For this review, take the finished solid that the model builds, in its own axes (mm). Face numbers are marked on the shaded views. Give positions to 0.01 mm unless a question says otherwise; leave off trailing zeros. Loops run counter-clockwise (first coordinate to the right, second up) from the corner with the lowest first, then second, coordinate; pieces in that order, holes last. Notation, with made-up numbers: M 30,82.25 L 65,82.25 A28 cw 65,105.25 Z; hole C 21,33.25 d5. An arc over 180 degrees is marked long. Use CSV: the item, a comma, the result in double quotes. Start each with the question number.
1. Take a section at C-C, the plane y = -357. Write out the cut boundary in (x, z).
2. To check wall thickness, follow line 1 (X direction, y = -164, z = 37.5); line 2 (X direction, y = -377.5, z = 65); line 3 (Y direction, x = -47.5, z = 100.5). State the ranges of each line that lie inside material, in increasing order. Write a range as [from, to].
3. Take a section at D-D, the plane x = -31. Write out the cut boundary in (y, z).
4. Take a section at B-B, the plane x = 20.5. Write out the cut boundary in (y, z).
5. Take a section at A-A, the plane z = 43. Write out the cut boundary in (x, y), and give its area (3 significant figures).
6. Insertion check: P1, Ø3, axis at x = -8.5, y = -187.5, coming from the +Z side; P2, Ø2, axis at y = -120.5, z = 373.5, coming from the -X side; P3, Ø5, axis at y = -248.5, z = 284, coming from the +X side. Each pin has a flat end and moves straight along its axis. Give the tip position at first contact, or say it passes through.
7. The part is to be moulded in two halves that separate along X. For the marked faces 1, 2, 3 and 4, say which applies: pulls with the +X half, pulls with the -X half, needs draft (parallel to the pull), parting line crosses it, or undercut.
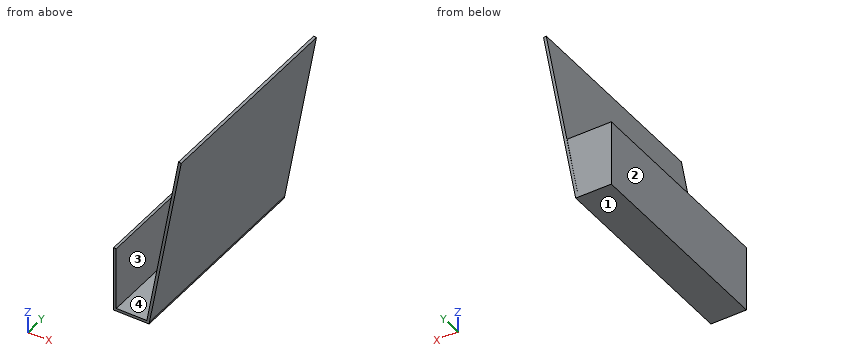
from build123d import *

# Parameters (mm, degrees)
F1_DEPTH = 482.6
F3_DEPTH = 6.35


with BuildPart() as f1:
    # F0 (on Front) → F1 (new body)
    with BuildSketch(Plane.XZ):
        Polygon((-69.85, 0), (0, 0), (1.085914, 6.158524), (0, 6.35), (-69.85, 6.35), align=None)
        Polygon((1.085914, 6.158524), (0, 0), (6.447959, 0), (7.339443, 5.055858), align=None)
        Polygon((74.981283, 425.239988), (1.085914, 6.158524), (7.339443, 5.055858), (81.234812, 424.137322), align=None)
        Polygon((-76.2, 0), (-69.85, 0), (-69.85, 6.35), (-69.85, 152.4), (-76.2, 152.4), align=None)
    extrude(amount=F1_DEPTH)

    # F2 (on Front) → F3 (join)
    with BuildSketch(Plane.XZ):
        Polygon((-76.2, 0), (0, 0), (26.39265, 152.4), (-76.2, 152.4), align=None)
    extrude(amount=F3_DEPTH)


solid = f1.part
Result set:
1,outline,"M -76.2,0 L 6.45,0 L 81.23,424.14 L 74.98,425.24 L 1.09,6.16 L 0,6.35 L -69.85,6.35 L -69.85,152.4 L -76.2,152.4 Z"
2,line 1,"[-76.2, -69.85], [6.61, 13.06]"
2,line 2,"[-76.2, -69.85], [11.46, 17.91]"
2,line 3,"[-6.35, 0]"
3,outline,"M -482.6,0 L 0,0 L 0,152.4 L -6.35,152.4 L -6.35,6.35 L -482.6,6.35 Z"
4,outline,"M -482.6,79.69 L 0,79.69 L 0,116.26 L -482.6,116.26 Z; M -6.35,118.37 L 0,118.37 L 0,152.4 L -6.35,152.4 Z"
5,outline,"M -76.2,-482.6 L -69.85,-482.6 L -69.85,-6.35 L 7.45,-6.35 L 7.45,0 L -76.2,0 Z; M 7.58,-482.6 L 14.03,-482.6 L 14.03,0 L 7.58,0 Z"
5,area,"6,670 mm2"
6,P1,"z = 6.35"
6,P2,"x = 65.68"
6,P3,"x = 56.97"
7,face 1,"needs draft"
7,face 2,"pulls with the -X half"
7,face 3,"undercut"
7,face 4,"undercut"
